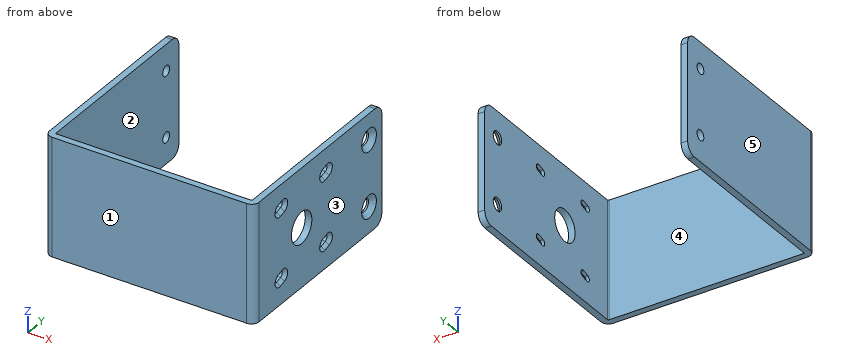
```python
from build123d import *

# Parameters (mm, degrees)
SKETCH5_W                                       = 160
SKETCH5_H                                       = 90
BASE_FLANGE1_DEPTH                              = 5
EDGE_FLANGE1_STRIP_W                            = 21.4732
EDGE_FLANGE1_STRIP_H                            = 5
EDGE_FLANGE1_STRIP_CUT_DEPTH                    = 90
EDGE_FLANGE1_STRIP_2_W                          = 21.4732
EDGE_FLANGE1_STRIP_2_H                          = 5
EDGE_FLANGE1_STRIP_CUT_2_DEPTH                  = 90
EDGE_FLANGE1_DEPTH                              = 90
EDGE_FLANGE1_BEND_DEPTH                         = 90
CUT_EXTRUDE1_REACH                              = 235.934
SKETCH16_R                                      = 12
SKETCH16_R_2                                    = 4
CUT_EXTRUDE2_REACH                              = 232.543
SKETCH20_R                                      = 4
CSK_FOR_M8_FLAT_HEAD_MACHINE_SCREW1_D           = 10
CSK_FOR_M8_FLAT_HEAD_MACHINE_SCREW1_DEPTH       = 10.25
CSK_FOR_M8_FLAT_HEAD_MACHINE_SCREW1_CSINK_D     = 17.3
CSK_FOR_M8_FLAT_HEAD_MACHINE_SCREW1_CSINK_ANGLE = 90
CSK_FOR_M8_FLAT_HEAD_MACHINE_SCREW1_TIP         = 3.004303095
BREAK_CORNER1_DEPTH                             = 160
CHAMFER2_SIZE                                   = 2.5


# Read off the part's stored shape, not the designer's step: Break-Corner1
# Sheet-metal steps are written as plain solids
with BuildPart() as part:
    # Sketch5 → Base-Flange1 (new body)
    with BuildSketch(Plane(origin=(0, 0, 0), x_dir=(1, 0, 0), z_dir=(0, 1, 0))):
        with Locations((80, 45)):
            Rectangle(SKETCH5_W, SKETCH5_H)
    extrude(amount=-BASE_FLANGE1_DEPTH)

    # Edge-Flange1 strip (across the edge) → Edge-Flange1 strip cut (cut)
    with BuildSketch(Plane.XY.offset(-90)):
        with Locations((-5, -2.5)):
            Rectangle(EDGE_FLANGE1_STRIP_W, EDGE_FLANGE1_STRIP_H)
    extrude(amount=EDGE_FLANGE1_STRIP_CUT_DEPTH, mode=Mode.SUBTRACT)

    # Edge-Flange1 strip 2 (across the edge) → Edge-Flange1 strip cut 2 (cut)
    with BuildSketch(Plane(origin=(160, 0, 0), x_dir=(-1, 0, 0), z_dir=(0, 0, -1))):
        with Locations((-5, -2.5)):
            Rectangle(EDGE_FLANGE1_STRIP_2_W, EDGE_FLANGE1_STRIP_2_H)
    extrude(amount=EDGE_FLANGE1_STRIP_CUT_2_DEPTH, mode=Mode.SUBTRACT)

    # Edge-Flange1 section (across the edge) → Edge-Flange1 (add)
    with BuildSketch(Plane.XY.offset(-90)):
        with BuildLine():
            Line((0, 0.7366), (0, 145))
            Line((0, 145), (5, 145))
            Line((5, 145), (5, 0.7366))
            ThreePointArc((5, 0.7366), (5.215745145, 0.215745145), (5.7366, 0))
            Line((5.7366, 0), (5.7366, -5))
            ThreePointArc((5.7366, -5), (1.680211239, -3.319788761), (0, 0.7366))
        make_face()
    extrude(amount=EDGE_FLANGE1_DEPTH)

    # Edge-Flange1 section 2 (across the edge) → Edge-Flange1 bend (add)
    with BuildSketch(Plane(origin=(160, 0, 0), x_dir=(-1, 0, 0), z_dir=(0, 0, -1))):
        with BuildLine():
            Line((0, 0.7366), (0, 145))
            Line((0, 145), (5, 145))
            Line((5, 145), (5, 0.7366))
            ThreePointArc((5, 0.7366), (5.215745145, 0.215745145), (5.7366, 0))
            Line((5.7366, 0), (5.7366, -5))
            ThreePointArc((5.7366, -5), (1.680211239, -3.319788761), (0, 0.7366))
        make_face()
    extrude(amount=EDGE_FLANGE1_BEND_DEPTH)

    # Sketch16 → Cut-Extrude1 (cut, up to next)
    with BuildSketch(Plane(origin=(160, 0, 0), x_dir=(0, 0, -1), z_dir=(1, 0, 0)), mode=Mode.PRIVATE) as cut_extrude1_sk1:
        with Locations(Location((45, 50.7366, 0), (0, 0, 90))):
            Circle(SKETCH16_R)
    cut_extrude1_tool1 = extrude(cut_extrude1_sk1.sketch, amount=-CUT_EXTRUDE1_REACH, mode=Mode.PRIVATE) & part.part
    # Sketch16 → Cut-Extrude1 (cut, up to next)
    with BuildSketch(Plane(origin=(160, 0, 0), x_dir=(0, 0, -1), z_dir=(1, 0, 0)), mode=Mode.PRIVATE) as cut_extrude1_sk2:
        with Locations(Location((20, 130, 0), (0, 0, 90))):
            Circle(SKETCH16_R_2)
    cut_extrude1_tool2 = extrude(cut_extrude1_sk2.sketch, amount=-CUT_EXTRUDE1_REACH, mode=Mode.PRIVATE) & part.part
    # Sketch16 → Cut-Extrude1 (cut, up to next)
    with BuildSketch(Plane(origin=(160, 0, 0), x_dir=(0, 0, -1), z_dir=(1, 0, 0)), mode=Mode.PRIVATE) as cut_extrude1_sk3:
        with Locations(Location((70, 130, 0), (0, 0, 270))):
            Circle(SKETCH16_R_2)
    cut_extrude1_tool3 = extrude(cut_extrude1_sk3.sketch, amount=-CUT_EXTRUDE1_REACH, mode=Mode.PRIVATE) & part.part
    # Sketch16 → Cut-Extrude1 (cut, up to next)
    with BuildSketch(Plane(origin=(160, 0, 0), x_dir=(0, 0, -1), z_dir=(1, 0, 0)), mode=Mode.PRIVATE) as cut_extrude1_sk4:
        with BuildLine():
            Line((16.334822748, 23.840907472), (15.043437692, 28.671261976))
            ThreePointArc((15.043437692, 28.671261976), (16.812922416, 31.732131756), (19.873792196, 29.962647032))
            Line((19.873792196, 29.962647032), (21.165177252, 25.132292528))
            ThreePointArc((21.165177252, 25.132292528), (19.395692528, 22.071422748), (16.334822748, 23.840907472))
        make_face()
    cut_extrude1_tool4 = extrude(cut_extrude1_sk4.sketch, amount=-CUT_EXTRUDE1_REACH, mode=Mode.PRIVATE) & part.part
    # Sketch16 → Cut-Extrude1 (cut, up to next)
    with BuildSketch(Plane(origin=(160, 0, 0), x_dir=(0, 0, -1), z_dir=(1, 0, 0)), mode=Mode.PRIVATE) as cut_extrude1_sk5:
        with BuildLine():
            Line((68.834822748, 23.840907472), (67.543437692, 28.671261976))
            ThreePointArc((67.543437692, 28.671261976), (69.312922416, 31.732131756), (72.373792196, 29.962647032))
            Line((72.373792196, 29.962647032), (73.665177252, 25.132292528))
            ThreePointArc((73.665177252, 25.132292528), (71.895692528, 22.071422748), (68.834822748, 23.840907472))
        make_face()
    cut_extrude1_tool5 = extrude(cut_extrude1_sk5.sketch, amount=-CUT_EXTRUDE1_REACH, mode=Mode.PRIVATE) & part.part
    # Sketch16 → Cut-Extrude1 (cut, up to next)
    with BuildSketch(Plane(origin=(160, 0, 0), x_dir=(0, 0, -1), z_dir=(1, 0, 0)), mode=Mode.PRIVATE) as cut_extrude1_sk6:
        with BuildLine():
            Line((16.334822748, 76.340907472), (15.043437692, 81.171261976))
            ThreePointArc((15.043437692, 81.171261976), (16.812922416, 84.232131756), (19.873792196, 82.462647032))
            Line((19.873792196, 82.462647032), (21.165177252, 77.632292528))
            ThreePointArc((21.165177252, 77.632292528), (19.395692528, 74.571422748), (16.334822748, 76.340907472))
        make_face()
    cut_extrude1_tool6 = extrude(cut_extrude1_sk6.sketch, amount=-CUT_EXTRUDE1_REACH, mode=Mode.PRIVATE) & part.part
    # Sketch16 → Cut-Extrude1 (cut, up to next)
    with BuildSketch(Plane(origin=(160, 0, 0), x_dir=(0, 0, -1), z_dir=(1, 0, 0)), mode=Mode.PRIVATE) as cut_extrude1_sk7:
        with BuildLine():
            Line((68.834822748, 76.340907472), (67.543437692, 81.171261976))
            ThreePointArc((67.543437692, 81.171261976), (69.312922416, 84.232131756), (72.373792196, 82.462647032))
            Line((72.373792196, 82.462647032), (73.665177252, 77.632292528))
            ThreePointArc((73.665177252, 77.632292528), (71.895692528, 74.571422748), (68.834822748, 76.340907472))
        make_face()
    cut_extrude1_tool7 = extrude(cut_extrude1_sk7.sketch, amount=-CUT_EXTRUDE1_REACH, mode=Mode.PRIVATE) & part.part
    add(cut_extrude1_tool1.solids().sort_by_distance((160, 50.7366, -45))[0], mode=Mode.SUBTRACT)
    add(cut_extrude1_tool2.solids().sort_by_distance((160, 130, -20))[0], mode=Mode.SUBTRACT)
    add(cut_extrude1_tool3.solids().sort_by_distance((160, 130, -70))[0], mode=Mode.SUBTRACT)
    add(cut_extrude1_tool4.solids().sort_by_distance((160, 26.901777, -18.104307))[0], mode=Mode.SUBTRACT)
    add(cut_extrude1_tool5.solids().sort_by_distance((160, 26.901777, -70.604307))[0], mode=Mode.SUBTRACT)
    add(cut_extrude1_tool6.solids().sort_by_distance((160, 79.401777, -18.104307))[0], mode=Mode.SUBTRACT)
    add(cut_extrude1_tool7.solids().sort_by_distance((160, 79.401777, -70.604307))[0], mode=Mode.SUBTRACT)

    # Sketch20 → Cut-Extrude2 (cut, up to next)
    with BuildSketch(Plane(origin=(5, 0, 0), x_dir=(0, 0, -1), z_dir=(1, 0, 0)), mode=Mode.PRIVATE) as cut_extrude2_sk1:
        with Locations(Location((70, 130, 0), (0, 0, 270))):
            Circle(SKETCH20_R)
    cut_extrude2_tool1 = extrude(cut_extrude2_sk1.sketch, amount=-CUT_EXTRUDE2_REACH, mode=Mode.PRIVATE) & part.part
    # Sketch20 → Cut-Extrude2 (cut, up to next)
    with BuildSketch(Plane(origin=(5, 0, 0), x_dir=(0, 0, -1), z_dir=(1, 0, 0)), mode=Mode.PRIVATE) as cut_extrude2_sk2:
        with Locations(Location((20, 130, 0), (0, 0, 90))):
            Circle(SKETCH20_R)
    cut_extrude2_tool2 = extrude(cut_extrude2_sk2.sketch, amount=-CUT_EXTRUDE2_REACH, mode=Mode.PRIVATE) & part.part
    add(cut_extrude2_tool1.solids().sort_by_distance((5, 130, -70))[0], mode=Mode.SUBTRACT)
    add(cut_extrude2_tool2.solids().sort_by_distance((5, 130, -20))[0], mode=Mode.SUBTRACT)

    # CSK for M8 Flat Head Machine Screw1
    with Locations(Plane(origin=(160, 0, 0), x_dir=(0, 0, -1), z_dir=(1, 0, 0))):
        with Locations((20, 130), (70, 130)):
            CounterSinkHole(CSK_FOR_M8_FLAT_HEAD_MACHINE_SCREW1_D / 2, CSK_FOR_M8_FLAT_HEAD_MACHINE_SCREW1_CSINK_D / 2, depth=CSK_FOR_M8_FLAT_HEAD_MACHINE_SCREW1_DEPTH, counter_sink_angle=CSK_FOR_M8_FLAT_HEAD_MACHINE_SCREW1_CSINK_ANGLE)
            with Locations((0, 0, -(CSK_FOR_M8_FLAT_HEAD_MACHINE_SCREW1_DEPTH + CSK_FOR_M8_FLAT_HEAD_MACHINE_SCREW1_TIP / 2))):  # 118° drill point
                Cone(0, CSK_FOR_M8_FLAT_HEAD_MACHINE_SCREW1_D / 2, CSK_FOR_M8_FLAT_HEAD_MACHINE_SCREW1_TIP, mode=Mode.SUBTRACT)

    # Break-Corner1 outline → Break-Corner1 (cut)
    with BuildSketch(Plane.YZ):
        with BuildLine():
            Line((145, -90), (145, -82))
            ThreePointArc((145, -82), (142.656854249, -87.656854249), (137, -90))
            Line((137, -90), (145, -90))
        make_face()
        with BuildLine():
            ThreePointArc((137, 0), (142.656854249, -2.343145751), (145, -8))
            Line((145, -8), (145, 0))
            Line((145, 0), (137, 0))
        make_face()
    extrude(amount=BREAK_CORNER1_DEPTH, mode=Mode.SUBTRACT)

    # Chamfer2
    chamfer2_edges = [part.edges().sort_by_distance(p)[0] for p in [
        (160, 22.071422748, -19.395692528),
        (160, 27.54746978, -20.519484724),
        (160, 31.732131756, -16.812922416),
        (160, 26.256084724, -15.68913022),
        (160, 22.071422748, -71.895692528),
        (160, 27.54746978, -73.019484724),
        (160, 31.732131756, -69.312922416),
        (160, 26.256084724, -68.18913022),
        (160, 74.571422748, -19.395692528),
        (160, 80.04746978, -20.519484724),
        (160, 84.232131756, -16.812922416),
        (160, 78.756084724, -15.68913022),
        (160, 74.571422748, -71.895692528),
        (160, 80.04746978, -73.019484724),
        (160, 84.232131756, -69.312922416),
        (160, 78.756084724, -68.18913022),
    ]]
    chamfer(chamfer2_edges, length=CHAMFER2_SIZE)


solid = part.part
```
Can you work these out from the model? Positions are in its coordinate system, mm. Face numbers are marked on the shaded views. A direction names the side the tool comes from. Coordinates: 2 decimals unless noted, no trailing zeros. Loops run counter-clockwise (first coordinate to the right, second up) from the corner with the lowest first, then second, coordinate; pieces in that order, holes last. Notation, with made-up numbers: (-1, 48) -> (56, 48) arc R21 ccw to (56, 52) -> close; hole circle Ø6 at (77, -25). An arc over 180 degrees is marked (long way). Put each result on its own line as item: value. Start each with the question number.
Q1. I'm going to push flat-ended pins straight in: P1, Ø9, axis at y = 130, z = -70, coming from the +X side; P2, Ø2, axis at x = 109, z = -47.5, coming from the +Y side; P3, Ø10.5, axis at y = 130, z = -20, coming from the +X side; P4, Ø6, axis at y = 130, z = -20, coming from the +X side. Where does each tip first touch, or does it pass through?
Q2. I want a section at D-D (x = 74.5). Write out the boundary of the cut face in (y, z), plus the area to 3 significant figures.
Q3. I want a section at B-B (z = -42). Write out the boundary of the cut face in (x, y), plus the area to 3 significant figures.
Q4. Thinking about a two-plate mould opening in X: for the marked faces 3, 4 and 5, which applies, pulls with the +X half, pulls with the -X half, needs draft (parallel to the pull), parting line crosses it, or undercut?
Q5. I want a section at C-C (y = 58.5). Write out the boundary of the cut face in (x, z).
Q6. If I drill on line 1 (Z direction, x = 1.7, y = 130); line 2 (Z direction, x = 155.4, y = 130); line 3 (X direction, y = 110.5, z = -15.5), over which ranges is the centre line in solid material (lowest first)? Write a range as [from, to].
Q7. I want a section at A-A (y = 130). Write out the boundary of the cut face in (x, z), plus the area to 3 significant figures.
Q8. For the marked faces 1 and 2, which set-ups out of +Z, -Z, +X, -X, +Y, -Y let a thin tool reach every point of the face, with its end or its side?
Taken from the geometry:
1. P1: stops at x = 5
1. P2: stops at y = 0
1. P3: stops at x = 156.6
1. P4: passes through
2. outline: (-5, -90) -> (0, -90) -> (0, 0) -> (-5, 0) -> close
2. area: 450 mm2
3. outline: (0, 0.74) arc R5.74 ccw to (5.74, -5) -> (154.26, -5) arc R5.74 ccw to (160, 0.74) -> (160, 39.12) -> (155, 39.12) -> (155, 0.74) arc R0.74 cw to (154.26, 0) -> (5.74, 0) arc R0.74 cw to (5, 0.74) -> (5, 145) -> (0, 145) -> close; (155, 62.36) -> (160, 62.36) -> (160, 145) -> (155, 145) -> close
3. area: 2,120 mm2
4. face 3: pulls with the +X half
4. face 4: undercut
4. face 5: pulls with the -X half
5. outline: (0, -90) -> (5, -90) -> (5, 0) -> (0, 0) -> close; (155, -90) -> (160, -90) -> (160, -54.15) -> (155, -54.15) -> close; (155, -35.85) -> (160, -35.85) -> (160, 0) -> (155, 0) -> close
6. line 1: z = [-90, -74], [-66, -24], [-16, 0]
6. line 2: z = [-90, -75], [-65, -25], [-15, 0]
6. line 3: x = [0, 5], [155, 160]
7. outline: (0, -90) -> (5, -90) -> (5, -74) -> (0, -74) -> close; (0, -66) -> (5, -66) -> (5, -24) -> (0, -24) -> close; (0, -16) -> (5, -16) -> (5, 0) -> (0, 0) -> close; (155, -90) -> (160, -90) -> (160, -78.65) -> (156.35, -75) -> (155, -75) -> close; (155, -65) -> (156.35, -65) -> (160, -61.35) -> (160, -28.65) -> (156.35, -25) -> (155, -25) -> close; (155, -15) -> (156.35, -15) -> (160, -11.35) -> (160, 0) -> (155, 0) -> close
7. area: 693 mm2
8. face 1: +Z, -Z, +X, -X, -Y
8. face 2: +Z, -Z, +Y
